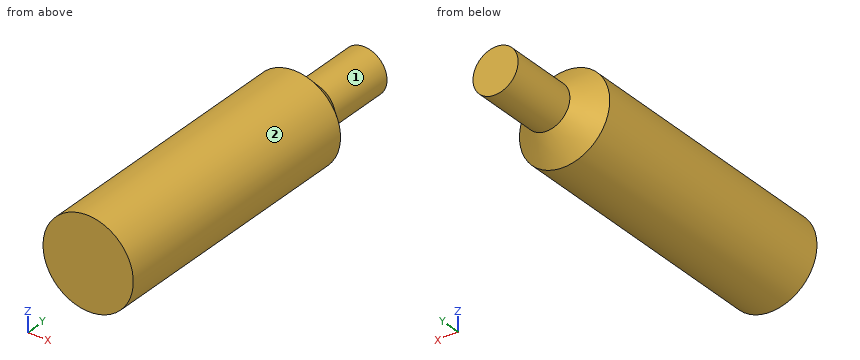
```python
from build123d import *

# Parameters (mm, degrees)
F0_W   = 12.7
F0_H   = 76.2
F0_W_2 = 6.35
F0_H_2 = 19.05


with BuildPart() as f1:
    # F0 (on Top) → F1 (revolve)
    with BuildSketch(Plane.XY):
        with Locations((-7.297987, -34.377149)):
            Rectangle(F0_W, F0_H)
    revolve(axis=Axis((-0.947987, -34.377149, 0), (0, 1, 0)))

    # F0 (on Top) → F2 (revolve)
    with BuildSketch(Plane.XY):
        Polygon((-7.297987, 10.072851), (-13.647987, 3.722851), (-0.947987, 3.722851), (-0.947987, 10.072851), align=None)
    revolve(axis=Axis((-0.947987, 16.422851, 0), (0, 1, 0)))

    # F0 (on Top) → F3 (revolve)
    with BuildSketch(Plane.XY):
        with Locations((-4.122987, 19.597851)):
            Rectangle(F0_W_2, F0_H_2)
    revolve(axis=Axis((-0.947987, 16.422851, 0), (0, 1, 0)))


solid = f1.part
```
The listing builds one solid part. Answer for the finished solid, in the listing's coordinates (mm). Face numbers are marked on the shaded views. A direction names the side the tool comes from. Coordinates: 2 decimals unless noted, no trailing zeros. Write each loop counter-clockwise with the first axis right and the second up, starting at its lowest first coordinate (ties: lowest second). Pieces come first, ordered by that corner, then holes. Notation, with made-up numbers: M -10.75,36.5 L 25.25,36.5 A26 ccw 25.25,51.5 Z; hole C -38.75,-35.75 d2. An arc over 180 degrees is marked long. Use a Markdown table: item, result. Add a question column.
1. Straight lines are drawn through the part: line 1 along Z through (x, y) = (-3.5, -33); line 2 along Y through (x, z) = (7.25, 9.5); line 3 along X through (y, z) = (13, 0.5). For each, find the intervals that lie inside material, in ascending order. Write a range as [from, to].
2. Which of the six approach directions +Z, -Z, +X, -X, +Y, -Y give full straight-line access (tool end or side, diameter ignored) to the marked faces 1 and 2?
3. Section C-C (y = -43.5) is taken. Give the vertices of the cut face in (x, z).
4. Section B-B (y = 19.5) is taken. Give the vertices of the cut face in (x, z).
5. Section A-A (z = 0) is taken. Give the vertices of the cut face in (x, y), plus the area to 3 significant figures.
6. Given P1, Ø5, axis at x = -4.5, y = -41.5, coming from the -Z side; P2, Ø1.5, axis at y = 6, z = 1.5, coming from the -X side; P3, Ø12, axis at x = -7.5, y = -51.5, coming from the +Z side, each flat-ended and moving along its own axis, determine where each tip first touches the part or whether it passes through.
Data:
| question | item | result |
|---|---|---|
| 1 | line 1 | z = [-12.44, 12.44] |
| 1 | line 2 | y = [-72.48, 3.87] |
| 1 | line 3 | x = [-7.28, 5.38] |
| 2 | face 1 | +Y |
| 2 | face 2 | +Y, -Y |
| 3 | outline | C -0.95,0 d25.4 |
| 4 | outline | C -0.95,0 d12.7 |
| 5 | outline | M -13.65,-72.48 L 11.75,-72.48 L 11.75,3.72 L 5.4,10.07 L 5.4,29.12 L -7.3,29.12 L -7.3,10.07 L -13.65,3.72 Z |
| 5 | area | 2,300 mm2 |
| 6 | P1 | stops at z = -12.66 |
| 6 | P2 | stops at x = -12.03 |
| 6 | P3 | stops at z = 12.69 |
